```python
from build123d import *

# Parameters (mm, degrees)
F0_W      = 200
F0_H      = 62
F1_DEPTH  = 15
F2_W      = 200
F2_H      = 62
F3_DEPTH  = 3
F4_W      = 5
F4_H      = 25
F5_DEPTH  = 7
F6_R      = 1.5
F7_DEPTH  = 12.6
F8_W      = 5
F8_H      = 25
F9_DEPTH  = 7
F10_R     = 1.5
F11_DEPTH = 25
F12_W     = 7
F12_H     = 4
F13_DEPTH = 20
F14_R     = 1.5
F15_DEPTH = 25
F16_W     = 7
F16_H     = 4
F17_DEPTH = 20
F18_R     = 1.5
F19_DEPTH = 25


with BuildPart() as f1:
    # F0 (on Front) → F1 (new body)
    with BuildSketch(Plane.XZ):
        Rectangle(F0_W, F0_H)
        Polygon((95, -24.5), (95, -26.5), (93, -26.5), (-93, -26.5), (-95, -26.5), (-95, -24.5), (-95, 24.5), (-95, 26.5), (-93, 26.5), (93, 26.5), (95, 26.5), (95, 24.5), align=None, mode=Mode.SUBTRACT)
        Polygon((-95, -26.5), (-93, -26.5), (-95, -24.5), align=None)
        Polygon((-95, 26.5), (-95, 24.5), (-93, 26.5), align=None)
        Polygon((93, -26.5), (95, -26.5), (95, -24.5), align=None)
        Polygon((93, 26.5), (95, 24.5), (95, 26.5), align=None)
    extrude(amount=F1_DEPTH)

    # F2 (on face) → F3 (join)
    with BuildSketch(Plane(origin=(0, 0, 0), x_dir=(-1, 0, 0), z_dir=(0, 1, 0))):
        Rectangle(F2_W, F2_H)
        Polygon((95, 24.5), (95, -24.5), (93, -26.5), (-93, -26.5), (-95, -24.5), (-95, 24.5), (-93, 26.5), (93, 26.5), align=None, mode=Mode.SUBTRACT)
        Polygon((93, -26.5), (95, -24.5), (95, 24.5), (93, 26.5), (-93, 26.5), (-95, 24.5), (-95, -24.5), (-93, -26.5), align=None)
    extrude(amount=F3_DEPTH)

    # F4 (on face) → F5 (join)
    with BuildSketch(Plane(origin=(-100, 0, 0), x_dir=(0, -1, 0), z_dir=(-1, 0, 0))):
        with Locations((-0.5, 12.5)):
            Rectangle(F4_W, F4_H)
        with Locations((-0.5, -12.5)):
            Rectangle(F4_W, F4_H)
    extrude(amount=F5_DEPTH)

    # F6 (on face) → F7 (cut)
    with BuildSketch(Plane.XZ.offset(2)):
        with Locations((-103.5, 12)):
            Circle(F6_R)
        with Locations((-103.5, 0)):
            Circle(F6_R)
        with Locations((-103.5, -12)):
            Circle(F6_R)
    extrude(amount=-F7_DEPTH, mode=Mode.SUBTRACT)

    # F8 (on face) → F9 (join)
    with BuildSketch(Plane.YZ.offset(100)):
        with Locations((0.5, 12.5)):
            Rectangle(F8_W, F8_H)
        with Locations((0.5, -12.5)):
            Rectangle(F8_W, F8_H)
    extrude(amount=F9_DEPTH)

    # F10 (on face) → F11 (cut)
    with BuildSketch(Plane.XZ.offset(2)):
        with Locations((103.6, 0)):
            Circle(F10_R)
        with Locations((103.6, 12)):
            Circle(F10_R)
        with Locations((103.6, -12)):
            Circle(F10_R)
    extrude(amount=-F11_DEPTH, mode=Mode.SUBTRACT)

    # F12 (on face) → F13 (join)
    with BuildSketch(Plane.XY.offset(31)):
        with Locations((-33.5, 1)):
            Rectangle(F12_W, F12_H)
        with Locations((33.5, 1)):
            Rectangle(F12_W, F12_H)
    extrude(amount=F13_DEPTH)

    # F14 (on face) → F15 (cut)
    with BuildSketch(Plane.XZ.offset(1)):
        with Locations((-33.5, 41)):
            Circle(F14_R)
        with Locations((33.5457399487, 41)):
            Circle(F14_R)
    extrude(amount=-F15_DEPTH, mode=Mode.SUBTRACT)

    # F16 (on face) → F17 (join)
    with BuildSketch(Plane(origin=(0, 0, -31), x_dir=(1, 0, 0), z_dir=(0, 0, -1))):
        with Locations((-33.5, -1)):
            Rectangle(F16_W, F16_H)
        with Locations((33.5, -1)):
            Rectangle(F16_W, F16_H)
    extrude(amount=F17_DEPTH)

    # F18 (on face) → F19 (cut)
    with BuildSketch(Plane.XZ.offset(1)):
        with Locations((-33.5, -41)):
            Circle(F18_R)
        with Locations((33.6346849799, -41)):
            Circle(F18_R)
    extrude(amount=-F19_DEPTH, mode=Mode.SUBTRACT)


solid = f1.part
```
CAD build for the part. Positions are in the model's coordinates, mm. A direction names the side the tool comes from. Round coordinates to 2 decimals unless told otherwise and drop trailing zeros. Order: outer loops, then holes, each group sorted by start corner. A loop starts at its lowest first (then second) coordinate and runs counter-clockwise, first axis right, second up. Notation, with made-up numbers: (-2.75, 78.25) - (24.25, 78.25) arc R26 cw to (24.25, 94.25) - close; hole circle Ø8 at (16, -23). An arc over 180 degrees is marked (long way). Answer as CSV lines item,"result". Start each with the question number.
1. Drill centre lines: L1, parallel to Z at x = -33.5, y = 2; L2, parallel to Z at x = 90.5, y = -3.25; L3, parallel to X at y = -3.25, z = 18.5. Where is each one in solid material? Low to high. Write a range as [from, to].
2. Saw through at B-B, the plane x = -8. Write the cut outline in (y, z), and give its area (3 significant figures).
3. Saw through at A-A, the plane y = -10. Write the cut outline in (x, z).
4. Pull direction Z, two halves, no side cores. Call faces 6 (the face through (101.9, -2, 0.3)), 7 (the face through (-103, 1, -25)), 8 (the face through (-103, 1, 25)), 9 (the face through (-95, -7, 0)): +Z half, -Z half, draft (parallel to the pull), parting line (faces both ways), or undercut.
5. Saw through at C-C, the plane z = -16.5. Write the cut outline in (x, y), and give its area (3 significant figures).
6. Pin check, flat tips, straight feed: pin 1 (4.5 mm diameter, centred on y = -5, z = -9.5, fed in from -X); pin 2 (9 mm diameter, centred on x = 14, y = -8, fed in from -Z); pin 3 (8 mm diameter, centred on x = -23.5, z = -7, fed in from -Y); pin 4 (2.5 mm diameter, centred on x = 103.6, z = -12, fed in from +Y). Stop position of each tip, or through.
7. Tool access for faces 1 (the face through (1, -7, -26.5)), 2 (the face through (-37, 1, 41)), 3 (the face through (103, 0, 25)), 4 (the face through (30, 1, 41)), 5 (the face through (-106, -2, 0)): list every direction of +Z, -Z, +X, -X, +Y, -Y with a clear straight run to the whole face (end or side of a thin tool).
Model answer:
1,L1,"z = [-51, -42.5], [-39.5, 39.5], [42.5, 51]"
1,L2,"z = [-31, -26.5], [26.5, 31]"
1,L3,"x = [-100, -95], [95, 100]"
2,outline,"(-15, -31) - (3, -31) - (3, 31) - (-15, 31) - (-15, 26.5) - (0, 26.5) - (0, -26.5) - (-15, -26.5) - close"
2,area,"321 mm²"
3,outline,"(-100, -31) - (100, -31) - (100, 31) - (-100, 31) - close; hole (-95, -24.5) - (-93, -26.5) - (93, -26.5) - (95, -24.5) - (95, 24.5) - (93, 26.5) - (-93, 26.5) - (-95, 24.5) - close"
4,face 6,"draft"
4,face 7,"-Z half"
4,face 8,"+Z half"
4,face 9,"undercut"
5,outline,"(-107, -2) - (-100, -2) - (-100, -15) - (-95, -15) - (-95, 0) - (95, 0) - (95, -15) - (100, -15) - (100, -2) - (107, -2) - (107, 3) - (-107, 3) - close"
5,area,"820 mm²"
6,pin 1,"stops at x = -100"
6,pin 2,"stops at z = -31"
6,pin 3,"stops at y = 0"
6,pin 4,"passes through"
7,face 1,"-Y"
7,face 2,"+Z, -X, +Y, -Y"
7,face 3,"+Z, +X, +Y, -Y"
7,face 4,"+Z, +Y, -Y"
7,face 5,"+Z, -Z, -X, -Y"
